Can you work these out from the drawing? Everything is in mm from the part's minimum corner. A direction names the side the tool comes from. Round coordinates to 2 decimals unless told otherwise and drop trailing zeros. Write each loop counter-clockwise with the first axis right and the second up, starting at its lowest first coordinate (ties: lowest second). Pieces come first, ordered by that corner, then holes. Notation, with made-up numbers: M 2,8 L 37,8 A22 ccw 37,35 Z; hole C 53.25,37.25 d5. An arc over 180 degrees is marked long. Answer in a Markdown table with one row per item. Add a question column.
(1) If I drill on probe 1 along Z at (x, y) = (27, 8.75); probe 2 along Y at (x, z) = (37, 1.75); probe 3 along Z at (x, y) = (10, 9.25), over which ranges is the centre line in solid material (lowest first)?
(2) For the marked faces 1 and 2, which set-ups out of +Z, -Z, +X, -X, +Y, -Y let a thin tool reach every point of the face, with its end or its side?
(3) Suppose I cut it at C-C, the plane y = 10. Write out the boundary of the cut face in (x, z).
(4) I'm going to push flat-ended pins straight in: pin 1 (6.5 mm diameter, centred on x = 10, z = 7, fed in from +Y); pin 2 (5 mm diameter, centred on y = 21.5, z = 3, fed in from -X); pin 3 (2.5 mm diameter, centred on x = 37, y = 5, fed in from -Z). Where does each tip first touch, or does it pass through?
(5) Suppose I cut it at B-B, the plane z = 12.75. Write out the boundary of the cut face in (x, y).
(6) Suppose I cut it at A-A, the plane x = 27. Write out the boundary of the cut face in (y, z), then the cut area to 3 significant figures.
(7) If we mould it in two halves opening along X, with no side actions, what happens to the marked faces 3, 4 and 5? For each: released by +X, released by -X, zero draft, split by the parting line, or undercut.
(8) Suppose I cut it at D-D, the plane x = 10. Write out the boundary of the cut face in (y, z).
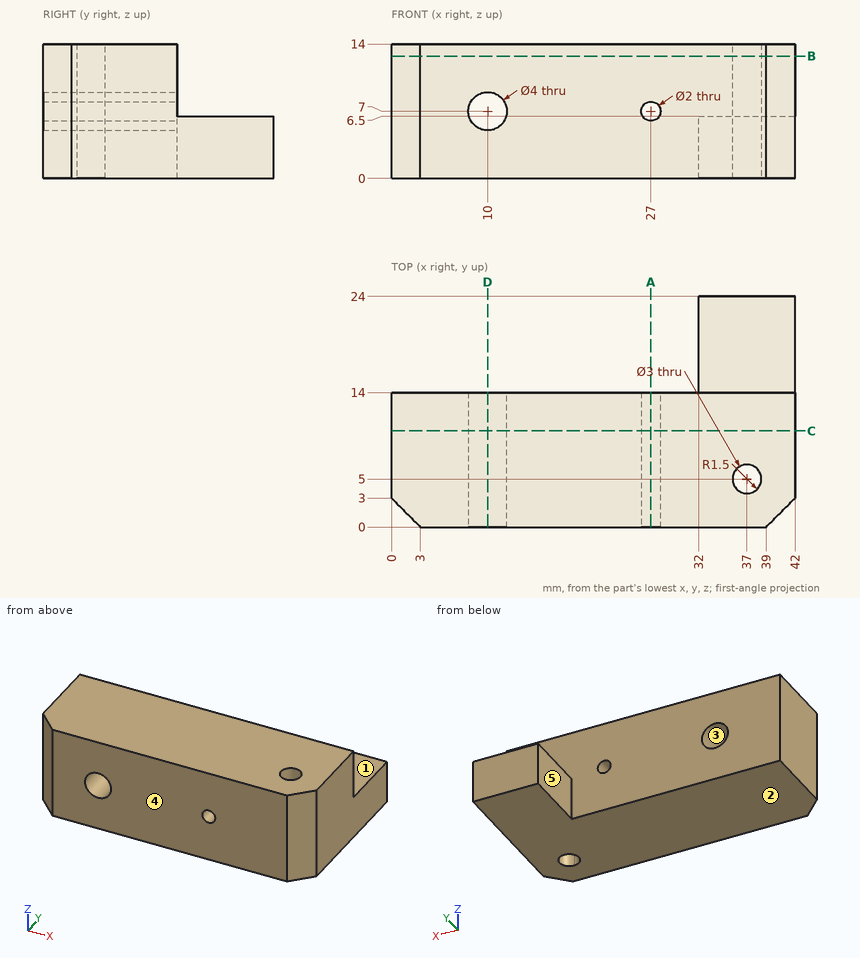
Calculated:
| question | item | result |
|---|---|---|
| 1 | probe 1 | 0 to 6, 8 to 14 |
| 1 | probe 2 | 0 to 3.5, 6.5 to 24 |
| 1 | probe 3 | 0 to 5, 9 to 14 |
| 2 | face 1 | +Z, +X, -X, +Y |
| 2 | face 2 | -Z, +X, -X, +Y, -Y |
| 3 | outline | M 0,0 L 42,0 L 42,14 L 0,14 Z; hole C 10,7 d4; hole C 27,7 d2 |
| 4 | pin 1 | y = 14 |
| 4 | pin 2 | x = 32 |
| 4 | pin 3 | through |
| 5 | outline | M 0,3 L 3,0 L 39,0 L 42,3 L 42,14 L 0,14 Z; hole C 37,5 d3 |
| 6 | outline | M 0,0 L 14,0 L 14,6 L 0,6 Z; M 0,8 L 14,8 L 14,14 L 0,14 Z |
| 6 | area | 168 mm² |
| 7 | face 3 | undercut |
| 7 | face 4 | zero draft |
| 7 | face 5 | released by -X |
| 8 | outline | M 0,0 L 14,0 L 14,5 L 0,5 Z; M 0,9 L 14,9 L 14,14 L 0,14 Z |
